Geometry: final body of the model. Coordinates: model frame, mm. A direction names the side the tool comes from. Coordinates: 2 decimals unless noted, no trailing zeros. Order: outer loops, then holes, each group sorted by start corner. A loop starts at its lowest first (then second) coordinate and runs counter-clockwise, first axis right, second up. Notation, with made-up numbers: M -1,38 L 24,38 A21 cw 24,44 Z; hole C 41,75.25 d3. An arc over 180 degrees is marked long. Use CSV: the item, a comma, the result in double quotes. Start each with the question number.
Q1. Section query A-A, the plane z = 0. Output: boundary loops of the cut face in (x, y).
Q2. Ray query, probe 1 along Z at (x, y) = (0, 3.8); probe 2 along Y at (x, z) = (10, -4.5); probe 3 along X at (y, z) = (3.75, -22.5). Return the intervals inside material, ascending.
Q3. First-contact query: P1, Ø1.5, axis at y = -1.5, z = 2.5, coming from the +X side; P2, Ø4, axis at x = 7, y = 1, coming from the +Z side; P3, Ø1.5, axis at y = -1.5, z = -4, coming from the -X side; P4, Ø2.5, axis at x = 0, z = 16.83, coming from the +Y side. Flat tips, straight axial feed; report the tip coordinate or a pass-through.
Q4. Access query for faces 4 (the face through (21, -1, -16.857)), 5 (the face through (-23.02, -1, 0)), 6 (the face through (-21, -1, 16.579)). Directions: +Z, -Z, +X, -X, +Y, -Y. A direction counts if a zero-diameter tool reaches every point of the face in a straight line with its end or side. Return the directions, or none.
Q5. Section query D-D, the plane z = -13. Output: boundary loops of the cut face in (x, y), and give its area (3 significant figures).
Q6. Mould query, pull axis X, two halves, no side actions, for faces 1 (the face through (21, -1, 16.857)), 2 (the face through (-9.088, 2.465, -40.924)), 3 (the face through (19.429, -1, 0)). Classes: +X half, -X half, draft (parallel to the pull), parting line (faces both ways), or undercut.
Q7. Section query B-B, the plane x = 0. Output: boundary loops of the cut face in (y, z).
Q8. Section query C-C, the plane y = -1. Output: boundary loops of the cut face in (x, z).
from build123d import *

# Parameters (mm, degrees)
F0_R     = 41.920471
F1_DEPTH = 5
F2_R     = 1.941315
F2_R_2   = 1.541244
F3_DEPTH = 50.7
F4_W     = 4
F4_H     = 33.157896
F4_H_2   = 33.714296
F6_DEPTH = 3


with BuildPart() as f1:
    # F0 (on Front) → F1 (new body)
    with BuildSketch(Plane.XZ):
        Circle(F0_R)
    extrude(amount=-F1_DEPTH)

    # F2 (on Front) → F3 (cut)
    with BuildSketch(Plane.XZ):
        with Locations((0, 16.827898)):
            Circle(F2_R)
        with Locations((0, -15.986843)):
            Circle(F2_R)
        Circle(F2_R_2)
    extrude(amount=-F3_DEPTH, mode=Mode.SUBTRACT)

    # F4 (on Front) → F6 (join)
    with BuildSketch(Plane.XZ):
        with Locations((-21.019738, 0)):
            Rectangle(F4_W, F4_H)
        with Locations((21.428579, 0)):
            Rectangle(F4_W, F4_H_2)
    extrude(amount=F6_DEPTH)


solid = f1.part
Responses:
1,outline,"M -41.92,0 L -23.02,0 L -23.02,-3 L -19.02,-3 L -19.02,0 L -1.54,0 L -1.54,5 L -41.92,5 Z; M 1.54,0 L 19.43,0 L 19.43,-3 L 23.43,-3 L 23.43,0 L 41.92,0 L 41.92,5 L 1.54,5 Z"
2,probe 1,"z = -41.92 to -17.93, -14.05 to -1.54, 1.54 to 14.89, 18.77 to 41.92"
2,probe 2,"y = 0 to 5"
2,probe 3,"x = -35.37 to 35.37"
3,P1,"stops at x = 23.43"
3,P2,"stops at z = 41.62"
3,P3,"stops at x = -23.02"
3,P4,"passes through"
4,face 4,"-Z, +X, -X, -Y"
4,face 5,"+Z, -Z, -X, -Y"
4,face 6,"+Z, -X, -Y"
5,outline,"M -39.85,0 L -23.02,0 L -23.02,-3 L -19.02,-3 L -19.02,0 L 19.43,0 L 19.43,-3 L 23.43,-3 L 23.43,0 L 39.85,0 L 39.85,5 L -39.85,5 Z"
5,area,"423 mm²"
6,face 1,"draft"
6,face 2,"parting line"
6,face 3,"undercut"
7,outline,"M 0,-41.92 L 5,-41.92 L 5,-17.93 L 0,-17.93 Z; M 0,-14.05 L 5,-14.05 L 5,-1.54 L 0,-1.54 Z; M 0,1.54 L 5,1.54 L 5,14.89 L 0,14.89 Z; M 0,18.77 L 5,18.77 L 5,41.92 L 0,41.92 Z"
8,outline,"M -23.02,-16.58 L -19.02,-16.58 L -19.02,16.58 L -23.02,16.58 Z; M 19.43,-16.86 L 23.43,-16.86 L 23.43,16.86 L 19.43,16.86 Z"
